CAD build for the part. Positions are in the model's coordinates, mm. A direction names the side the tool comes from. Give positions to 0.01 mm unless a question says otherwise; leave off trailing zeros. Loops run counter-clockwise (first coordinate to the right, second up) from the corner with the lowest first, then second, coordinate; pieces in that order, holes last.
```python
from build123d import *

# Parameters (mm, degrees)
SKETCH1_R           = 14.605
BOSS_EXTRUDE1_DEPTH = 25.4
SKETCH2_R           = 16.51
BOSS_EXTRUDE2_DEPTH = 63.5
SKETCH5_R           = 13.462
CUT_EXTRUDE1_DEPTH  = 24.13
SKETCH6_R           = 15.24
CUT_EXTRUDE3_DEPTH  = 60.96
CUT_EXTRUDE4_REACH  = 67.278
SKETCH7_R           = 6.35
SKETCH9_W           = 7.62
SKETCH9_H           = 44.45
CUT_EXTRUDE5_DEPTH  = 92.915016183
CIRPATTERN1_COUNT   = 3
SKETCH10_R          = 20.32
SKETCH10_R_2        = 15.24
BOSS_EXTRUDE3_DEPTH = 2.54
SKETCH11_R          = 21.59
SKETCH11_R_2        = 20.32
BOSS_EXTRUDE4_DEPTH = 15.24
SKETCH12_R          = 21.59
SKETCH12_R_2        = 20.32
BOSS_EXTRUDE5_DEPTH = 2.54


with BuildPart() as part:
    # Sketch1 → Boss-Extrude1 (new body)
    with BuildSketch(Plane.XY):
        Circle(SKETCH1_R)
    extrude(amount=BOSS_EXTRUDE1_DEPTH)

    # Sketch2 → Boss-Extrude2 (add)
    with BuildSketch(Plane.XY.offset(25.4)):
        Circle(SKETCH2_R)
    extrude(amount=BOSS_EXTRUDE2_DEPTH)

    # Sketch5 → Cut-Extrude1 (cut)
    with BuildSketch(Plane(origin=(0, 0, 0), x_dir=(-1, 0, 0), z_dir=(0, 0, -1))):
        Circle(SKETCH5_R)
    extrude(amount=-CUT_EXTRUDE1_DEPTH, mode=Mode.SUBTRACT)

    # Sketch6 → Cut-Extrude3 (cut)
    with BuildSketch(Plane.XY.offset(88.9)):
        Circle(SKETCH6_R)
    extrude(amount=-CUT_EXTRUDE3_DEPTH, mode=Mode.SUBTRACT)

    # Sketch7 → Cut-Extrude4 (cut, up to next)
    with BuildSketch(Plane.XY.offset(27.94), mode=Mode.PRIVATE) as cut_extrude4_sk1:
        Circle(SKETCH7_R)
    cut_extrude4_tool1 = extrude(cut_extrude4_sk1.sketch, amount=-CUT_EXTRUDE4_REACH, mode=Mode.PRIVATE) & part.part
    add(cut_extrude4_tool1.solids().sort_by_distance((0, 0, 27.94))[0], mode=Mode.SUBTRACT)

    # Sketch9 → Cut-Extrude5 (cut, symmetric)
    with BuildSketch(Plane(origin=(0, 0, 0), x_dir=(1, 0, 0), z_dir=(0, 1, 0))):
        with Locations((0, -60.325)):
            Rectangle(SKETCH9_W, SKETCH9_H)
    cut_extrude5 = extrude(amount=CUT_EXTRUDE5_DEPTH, both=True, mode=Mode.SUBTRACT)

    # CirPattern1: Cut-Extrude5 ×3 about axis
    cirpattern1_axis = Axis((0, 0, 0), (0, 0, 1))
    for i in range(1, CIRPATTERN1_COUNT):
        add(cut_extrude5.rotate(cirpattern1_axis, i * 360 / CIRPATTERN1_COUNT), mode=Mode.SUBTRACT)



with BuildPart() as body_2:
    # Sketch10 → Boss-Extrude3 (new body)
    with BuildSketch(Plane.XY.offset(88.9)):
        Circle(SKETCH10_R)
        Circle(SKETCH10_R_2, mode=Mode.SUBTRACT)
    extrude(amount=BOSS_EXTRUDE3_DEPTH)


with BuildPart() as body_3:
    # Sketch11 → Boss-Extrude4 (new body)
    with BuildSketch(Plane.XY.offset(91.44)):
        with Locations(Location((0, 0, 0), (0, 0, 180))):
            Circle(SKETCH11_R)
        with Locations(Location((0, 0, 0), (0, 0, 180))):
            Circle(SKETCH11_R_2, mode=Mode.SUBTRACT)
    extrude(amount=BOSS_EXTRUDE4_DEPTH)


with BuildPart() as part_1:
    add(part.part)

    add(body_2.part)  # Boss-Extrude5 merges body 2

    add(body_3.part)  # Boss-Extrude5 merges body 3
    # Sketch12 → Boss-Extrude5 (add)
    with BuildSketch(Plane(origin=(0, 0, 91.44), x_dir=(-1, 0, 0), z_dir=(0, 0, -1))):
        with Locations(Location((0, 0, 0), (0, 0, 180))):
            Circle(SKETCH12_R)
        Circle(SKETCH12_R_2, mode=Mode.SUBTRACT)
    extrude(amount=BOSS_EXTRUDE5_DEPTH)


solid = part_1.part
```
1. Tool access for faces 1 (the face through (-10.764, 9.871, 12.522)), 2 (the face through (2.92, 15.15, 91.44)), 3 (the face through (-1.38, -6.2, 26.06)): list every direction of +Z, -Z, +X, -X, +Y, -Y with a clear straight run to the whole face (end or side of a thin tool).
Responses:
face 1: -Z
face 2: +Z
face 3: +Z, -Z
2. Pull direction X, two halves, no side cores. Call faces 4 (the face through (-16, 13, 106.68)), 5 (the face through (10.683, -8.191, 11.896)), 6 (the face through (8.88, 13.92, 56.71)): released by +X, released by -X, zero draft, split by the parting line, or undercut.
Responses:
face 4: zero draft
face 5: undercut
face 6: split by the parting line
3. Drop flat-ended pins along their axis: pin 1 (10 mm diameter, centred on x = -14, y = 4.5, fed in from -Z); pin 2 (1 mm diameter, centred on y = -15, z = 70.5, fed in from -X); pin 3 (1.4 mm diameter, centred on x = -1, y = 16, fed in from +Z); pin 4 (1 mm diameter, centred on x = -1.5, z = 32, fed in from +Y). Give the stop position or say it passes through.
Responses:
pin 1: stops at z = 0
pin 2: stops at x = -7.89
pin 3: stops at z = 91.44
pin 4: stops at y = 16.48
4. Saw through at A-A, the plane y = 0. List the corners of the cut face in (x, z) (3 decimals), and give its area (3 significant figures).
Responses:
outline: (-21.59, 88.9) - (-16.51, 88.9) - (-16.51, 25.4) - (-14.605, 25.4) - (-14.605, 0) - (-13.462, 0) - (-13.462, 24.13) - (-6.35, 24.13) - (-6.35, 27.94) - (-15.24, 27.94) - (-15.24, 91.44) - (-20.32, 91.44) - (-20.32, 106.68) - (-21.59, 106.68) - close; (6.35, 24.13) - (13.462, 24.13) - (13.462, 0) - (14.605, 0) - (14.605, 25.4) - (16.51, 25.4) - (16.51, 88.9) - (21.59, 88.9) - (21.59, 106.68) - (20.32, 106.68) - (20.32, 91.44) - (15.24, 91.44) - (15.24, 27.94) - (6.35, 27.94) - close
area: 354 mm2
5. Saw through at C-C, the plane y = -9. Count the separate pieces of the cut face and the enclosed holes in it, and give its area (3 significant figures).
Responses:
separate pieces: 3
enclosed holes: 0
area: 303 mm2
6. Probe line 1 along Y through (x, z) = (0, 96); line 2 along Y through (x, z) = (0, 25) (3 decimals); line 3 along Z through (x, y) = (3.5, -5.5). List the from-to ranges inside material, lowest first.
Responses:
line 1: y = -21.59 to -20.32, 20.32 to 21.59
line 2: y = -14.605 to -6.35, 6.35 to 14.605
line 3: z = 24.13 to 27.94
7. Saw through at B-B, the plane z = 71.5. List the corners of the cut face in (x, y), and give its area (3 significant figures).
Responses:
outline: (-15.82, -4.73) - (-14.68, -4.08) arc R15.24 cw to (-14.68, 4.08) - (-15.82, 4.73) arc R16.51 ccw to start; (-12.01, -11.33) arc R16.51 ccw to (-3.81, -16.06) - (-3.81, -14.76) arc R15.24 cw to (-10.87, -10.68) - close; (-12.01, 11.33) - (-10.87, 10.68) arc R15.24 cw to (-3.81, 14.76) - (-3.81, 16.06) arc R16.51 ccw to start; (3.81, -16.06) arc R16.51 ccw to (12.01, -11.33) - (10.87, -10.68) arc R15.24 cw to (3.81, -14.76) - close; (3.81, 14.76) arc R15.24 cw to (10.87, 10.68) - (12.01, 11.33) arc R16.51 ccw to (3.81, 16.06) - close; (14.68, -4.08) - (15.82, -4.73) arc R16.51 ccw to (15.82, 4.73) - (14.68, 4.08) arc R15.24 cw to start
area: 68.0 mm2
